Input: part model. Units: mm. Frame: model coordinates. A direction names the side the tool comes from. Coordinates: 2 decimals unless noted, no trailing zeros. Answer in a Markdown table with one row per item.
from build123d import *

# Parameters (mm, degrees)
SKETCH_1_R          = 26
SKETCH_1_R_2        = 5
SKETCH_1_R_3        = 1.7
SKETCH_1_R_4        = 1.45
EXTRUDE_1_DEPTH     = 4
SKETCH_2_R          = 14
SKETCH_2_R_2        = 12
CUT_EXTRUDE_1_DEPTH = 0.2
SKETCH_3_R          = 14
SKETCH_3_R_2        = 12
CUT_EXTRUDE_2_DEPTH = 0.2
SKETCH_5_R          = 27.923918385
SKETCH_5_R_2        = 25.46843451
CUT_EXTRUDE_3_DEPTH = 1.25
CHAMFER_1_SIZE      = 0.2
FILLET_1_R          = 0.2
SKETCH_6_R          = 3.25
CUT_EXTRUDE_4_DEPTH = 3.3


with BuildPart() as part:
    # 草图1 → 凸台-拉伸1 (new body, symmetric)
    with BuildSketch(Plane(origin=(0, 0, 0), x_dir=(1, 0, 0), z_dir=(0, 1, 0))):
        Circle(SKETCH_1_R)
        Circle(SKETCH_1_R_2, mode=Mode.SUBTRACT)
        with Locations((-10.5, 18.186533479)):
            Circle(SKETCH_1_R_3, mode=Mode.SUBTRACT)
        with Locations((10.5, 18.186533479)):
            Circle(SKETCH_1_R_3, mode=Mode.SUBTRACT)
        with Locations((21, 0)):
            Circle(SKETCH_1_R_3, mode=Mode.SUBTRACT)
        with Locations((10.5, -18.186533479)):
            Circle(SKETCH_1_R_3, mode=Mode.SUBTRACT)
        with Locations((-10.5, -18.186533479)):
            Circle(SKETCH_1_R_3, mode=Mode.SUBTRACT)
        with Locations((-21, 0)):
            Circle(SKETCH_1_R_3, mode=Mode.SUBTRACT)
        with Locations((0, 8)):
            Circle(SKETCH_1_R_4, mode=Mode.SUBTRACT)
        with Locations((8, 0)):
            Circle(SKETCH_1_R_4, mode=Mode.SUBTRACT)
        with Locations((0, -8)):
            Circle(SKETCH_1_R_4, mode=Mode.SUBTRACT)
        with Locations((-8, 0)):
            Circle(SKETCH_1_R_4, mode=Mode.SUBTRACT)
    extrude(amount=EXTRUDE_1_DEPTH, both=True)

    # 草图2 → 切除-拉伸1 (cut)
    with BuildSketch(Plane(origin=(0, 4, 0), x_dir=(1, 0, 0), z_dir=(0, 1, 0))):
        Circle(SKETCH_2_R)
        Circle(SKETCH_2_R_2, mode=Mode.SUBTRACT)
    extrude(amount=-CUT_EXTRUDE_1_DEPTH, mode=Mode.SUBTRACT)

    # 草图3 → 切除-拉伸2 (cut)
    with BuildSketch(Plane.XZ.offset(4)):
        Circle(SKETCH_3_R)
        Circle(SKETCH_3_R_2, mode=Mode.SUBTRACT)
    extrude(amount=-CUT_EXTRUDE_2_DEPTH, mode=Mode.SUBTRACT)

    # 草图5 → 切除-拉伸3 (cut, symmetric)
    with BuildSketch(Plane(origin=(0, 0, 0), x_dir=(1, 0, 0), z_dir=(0, 1, 0))):
        Circle(SKETCH_5_R)
        Circle(SKETCH_5_R_2, mode=Mode.SUBTRACT)
    extrude(amount=CUT_EXTRUDE_3_DEPTH, both=True, mode=Mode.SUBTRACT)

    # 倒角1
    chamfer_1_edges = [part.edges().sort_by_distance(p)[0] for p in [
        (-26, 1.25, 0),
        (-26, -1.25, 0),
    ]]
    chamfer(chamfer_1_edges, length=CHAMFER_1_SIZE)

    # 圆角1
    fillet_1_edges = [part.edges().sort_by_distance(p)[0] for p in [
        (-26, -4, 0),
        (-26, 4, 0),
        (-5, -4, 0),
        (-5, 4, 0),
    ]]
    fillet(fillet_1_edges, radius=FILLET_1_R)

    # 草图6 → 切除-拉伸4 (cut)
    with BuildSketch(Plane.XZ.offset(4)):
        with Locations((-21, 0)):
            Circle(SKETCH_6_R)
        with Locations((-10.5, -18.186533479)):
            Circle(SKETCH_6_R)
        with Locations((10.5, -18.186533479)):
            Circle(SKETCH_6_R)
        with Locations((21, 0)):
            Circle(SKETCH_6_R)
        with Locations((10.5, 18.186533479)):
            Circle(SKETCH_6_R)
        with Locations((-10.5, 18.186533479)):
            Circle(SKETCH_6_R)
    extrude(amount=-CUT_EXTRUDE_4_DEPTH, mode=Mode.SUBTRACT)


solid = part.part
1) Cut plane A-A, the plane x = 0. State how many separate pieces and enclosed holes the cut face has, and give its area (3 significant figures).
Resolved:
| item | result |
|---|---|
| separate pieces | 4 |
| enclosed holes | 0 |
| area | 285 mm2 |
2) Contact query for flat-ended pins moving along their axis: pin 1 (2 mm diameter, centred on x = -9.5, z = 18.5, fed in from -Y); pin 2 (2 mm diameter, centred on x = 10.5, z = -18.19, fed in from +Y); pin 3 (3 mm diameter, centred on y = -1.5, z = 19.5, fed in from +X); pin 4 (2 mm diameter, centred on x = 13.5, y = 1.5, fed in from -Z). Output: stop coordinate, or through.
Resolved:
| item | result |
|---|---|
| pin 1 | stops at y = -0.7 |
| pin 2 | passes through |
| pin 3 | stops at x = 18.76 |
| pin 4 | stops at z = -22.8 |
3) Reachability of faces 1 (the face through (-13.747, -2.373, 18.329)), 2 (the face through (-9.45, -0.06, -0.06)) from +Z, -Z, +X, -X, +Y, -Y: full face, straight path, thin tool, end or side. Return the list, or none.
Resolved:
| item | result |
|---|---|
| face 1 | -Y |
| face 2 | +Y, -Y |
4) Material intervals for probe 1 along Z at (x, y) = (10.5, -2.5); probe 2 along X at (y, z) = (3.75, -1); probe 3 along X at (y, z) = (-1.75, -20), sorted ascending.
Resolved:
| item | result |
|---|---|
| probe 1 | z = -23.79 to -21.44, -14.94 to 14.94, 21.44 to 23.79 |
| probe 2 | x = -25.98 to -22.37, -19.63 to -9.05, -6.95 to -4.9, 4.9 to 6.95, 9.05 to 19.63, 22.37 to 25.98 |
| probe 3 | x = -16.61 to -13.2, -7.8 to 7.8, 13.2 to 16.61 |
